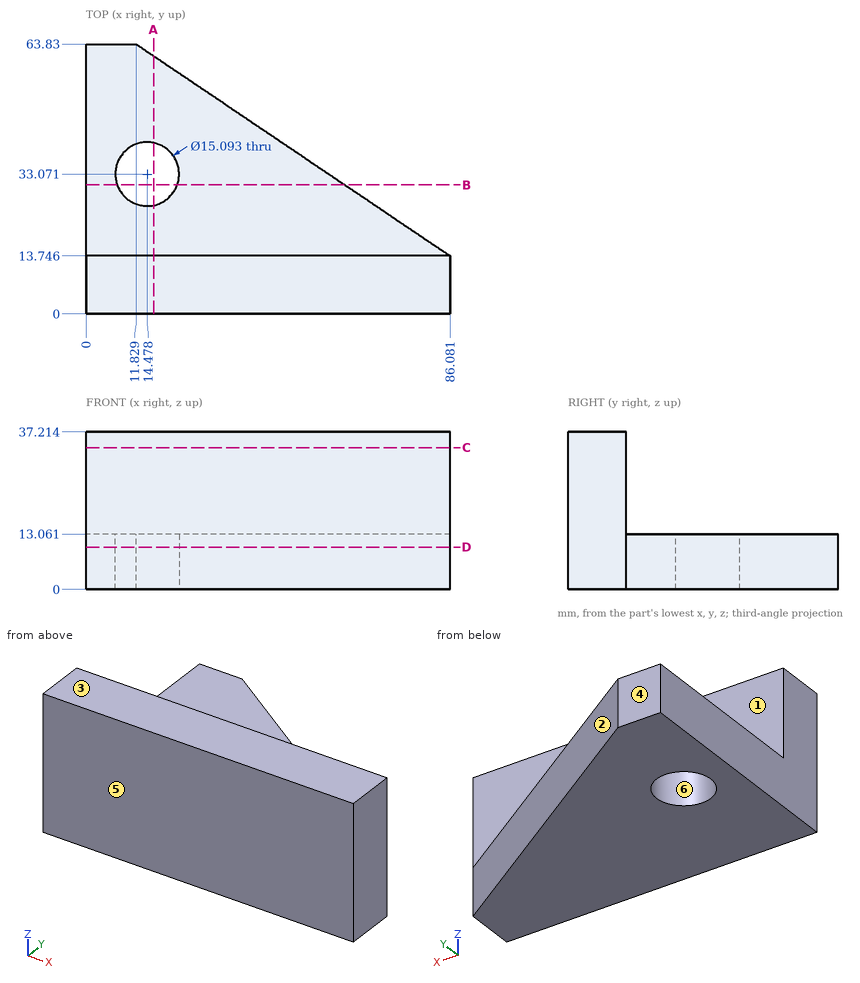
For this review, use the dimensioned drawing (mm, ordinates from the lowest corner) and the shaded views. A direction names the side the tool comes from. Coordinates: 2 decimals unless noted, no trailing zeros. Loops run counter-clockwise (first coordinate to the right, second up) from the corner with the lowest first, then second, coordinate; pieces in that order, holes last.
1. Insertion check: P1, Ø5, axis at x = 51, z = 10.5, coming from the +Y side (1 decimal); P2, Ø5, axis at y = 39.5, z = 10.5, coming from the +X side (1 decimal); P3, Ø12, axis at x = 26.5, z = 29.5, coming from the +Y side. Each pin has a flat end and moves straight along its axis. Give the tip position at first contact, or say it passes through.
2. Add section D-D, the plane z = 10. Give the boundary of the cut face in (x, y) (1 decimal).
3. Mouldability with a two-part tool opening along Y and no side actions: class the marked faces 3, 4, 5 and 6 as +Y half, -Y half, draft (parallel to the pull), parting line (faces both ways), or undercut.
4. Add section B-B, the plane y = 30.5. Give the boundary of the cut face in (x, z).
5. Add section C-C, the plane z = 33.5. Give the boundary of the cut face in (x, y), then the cut area to 3 significant figures.
6. For line 1 (Z direction, x = 31, y = 32); line 2 (X direction, y = 35.5, z = 3.5) (1 decimal); line 3 (Y direction, x = 74.5, z = 18.5), list the stretches that pass through material, from the lowest coordinate up.
7. Add section A-A, the plane x = 16. Give the boundary of the cut face in (y, z), then the cut area to 3 significant figures.
8. For the marked faces 1 and 2, list the 3-axis set-ups (+Z, -Z, +X, -X, +Y, -Y) from which the entire face can be reached by the end or side of a thin tool; tool diameter is ignored.
Result:
1. P1: stops at y = 39.1
1. P2: stops at x = 51.6
1. P3: stops at y = 13.75
2. outline: (0, 0) - (86.1, 0) - (86.1, 13.7) - (11.8, 63.8) - (0, 63.8) - close; hole circle Ø15.1 at (14.5, 33.1)
3. face 3: draft
3. face 4: +Y half
3. face 5: -Y half
3. face 6: undercut
4. outline: (0, 0) - (7.38, 0) - (7.38, 13.06) - (0, 13.06) - close; (21.57, 0) - (61.24, 0) - (61.24, 13.06) - (21.57, 13.06) - close
5. outline: (0, 0) - (86.08, 0) - (86.08, 13.75) - (0, 13.75) - close
5. area: 1,180 mm2
6. line 1: z = 0 to 13.06
6. line 2: x = 0 to 7.3, 21.6 to 53.8
6. line 3: y = 0 to 13.75
7. outline: (0, 0) - (25.68, 0) - (25.68, 13.06) - (13.75, 13.06) - (13.75, 37.21) - (0, 37.21) - close; (40.46, 0) - (61.02, 0) - (61.02, 13.06) - (40.46, 13.06) - close
7. area: 936 mm2
8. face 1: +Z, +X, -X, +Y
8. face 2: +Z, -Z, +X, +Y
